Can you work these out from the drawing? Everything is in mm from the part's minimum corner. Round coordinates to 2 decimals unless told otherwise and drop trailing zeros. Loops run counter-clockwise (first coordinate to the right, second up) from the corner with the lowest first, then second, coordinate; pieces in that order, holes last. Notation, with made-up numbers: (-32, 64.5) -> (6, 64.5) arc R25 cw to (6, 103.5) -> close; hole circle Ø4 at (-20, 87.25). An arc over 180 degrees is marked (long way). Answer as a JSON object with one key per item and string values.
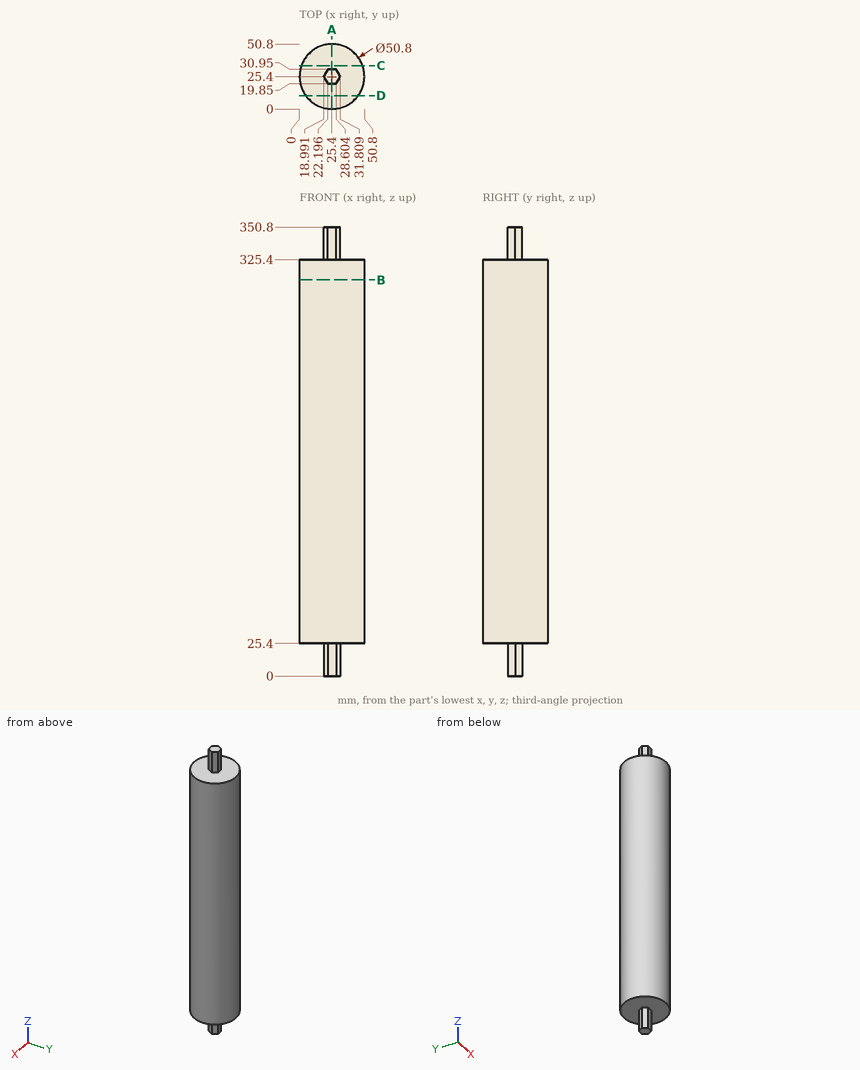
Q1. I want a section at B-B, the plane z = 309.5. Write out the boundary of the cut face in (x, y).
Determined:
{"outline": "circle Ø50.8 at (25.4, 25.4)"}
Q2. I want a section at A-A, the plane x = 25.4. Write out the boundary of the cut face in (y, z), then the cut area to 3 significant figures.
Determined:
{"outline": "(0, 25.4) -> (19.85, 25.4) -> (19.85, 0) -> (30.95, 0) -> (30.95, 25.4) -> (50.8, 25.4) -> (50.8, 325.4) -> (30.95, 325.4) -> (30.95, 350.8) -> (19.85, 350.8) -> (19.85, 325.4) -> (0, 325.4) -> close", "area": "15,800 mm²"}
Q3. I want a section at D-D, the plane y = 10.5. Write out the boundary of the cut face in (x, z).
Determined:
{"outline": "(4.83, 25.4) -> (45.97, 25.4) -> (45.97, 325.4) -> (4.83, 325.4) -> close"}
Q4. I'm going to push flat-ended pins straight in: pin 1 (12 mm diameter, centred on x = 35, z = 159, fed in from -Y); pin 2 (6 mm diameter, centred on y = 12, z = 229.5, fed in from +X); pin 3 (3 mm diameter, centred on x = 25, z = 335.5, fed in from +Y). Where does each tip first touch, or does it pass through?
Determined:
{"pin 1": "y = 0.26", "pin 2": "x = 48.57", "pin 3": "y = 30.95"}
Q5. If I drill on L1, parallel to Z at x = 15, y = 32.5; L2, parallel to Y at x = 25.5, z = 249.5; L3, parallel to Y at x = 23.5, z = 58.5, over which ranges is the centre line in solid material (lowest first)? Write a range as [from, to].
Determined:
{"L1": "[25.4, 325.4]", "L2": "[0, 50.8]", "L3": "[0.07, 50.73]"}
Q6. I want a section at C-C, the plane y = 34. Write out the boundary of the cut face in (x, z), then the cut area to 3 significant figures.
Determined:
{"outline": "(1.5, 25.4) -> (49.3, 25.4) -> (49.3, 325.4) -> (1.5, 325.4) -> close", "area": "14,300 mm²"}
